CAD build for the part. Positions are in the model's coordinates, mm. Give positions to 0.01 mm unless a question says otherwise; leave off trailing zeros. Order: outer loops, then holes, each group sorted by start corner. A loop starts at its lowest first (then second) coordinate and runs counter-clockwise, first axis right, second up.
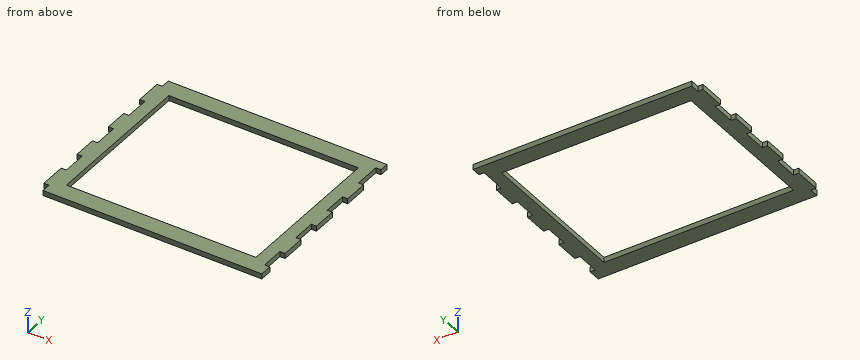
Autodesk Inventor part; units mm, degrees
ref_plane "YZ Plane" through (0, 0, 0) normal (1, 0, 0) x (0, 1, 0)
ref_plane "XZ Plane" through (0, 0, 0) normal (0, 1, 0) x (-1, 0, 0)
ref_plane "XY Plane" through (0, 0, 0) normal (0, 0, 1) x (1, 0, 0)
sketch "Boceto1" plane through (0, 0, 0) normal (0, 0, 1) x (1, 0, 0)
  line L0 (3, 3) -> (130, 3)
  line L1 (10, 103) -> (10, 13)
  line L2 (10, 13) -> (120, 13)
  line L3 (120, 13) -> (120, 103)
  line L4 (10, 103) -> (120, 103)
  line L5 (130, 113) -> (130, 106)
  line L6 (130, 106) -> (127, 107.7321)
  line L7 (130, 92.5) -> (127, 90.7679)
  line L8 (130, 65) -> (127, 63.2679)
  line L9 (130, 78.5) -> (127, 80.2321)
  line L10 (130, 10) -> (127, 8.2679)
  line L11 (130, 23.5) -> (127, 25.2321)
  line L12 (130, 51) -> (127, 52.7321)
  line L13 (130, 37.5) -> (127, 35.7679)
  line L14 (127, 107.7321) -> (127, 90.7679)
  line L15 (127, 80.2321) -> (127, 63.2679)
  line L16 (127, 52.7321) -> (127, 35.7679)
  line L17 (127, 25.2321) -> (127, 8.2679)
  line L18 (3, 113) -> (3, 106)
  line L19 (3, 106) -> (0, 107.7321)
  line L20 (3, 92.5) -> (0, 90.7679)
  line L21 (3, 65) -> (0, 63.2679)
  line L22 (3, 78.5) -> (0, 80.2321)
  line L23 (3, 10) -> (0, 8.2679)
  line L24 (3, 23.5) -> (0, 25.2321)
  line L25 (3, 37.5) -> (0, 35.7679)
  line L26 (3, 51) -> (0, 52.7321)
  line L27 (0, 107.7321) -> (0, 90.7679)
  line L28 (0, 80.2321) -> (0, 63.2679)
  line L29 (0, 52.7321) -> (0, 35.7679)
  line L30 (0, 25.2321) -> (0, 8.2679)
  line L31 (130, 113) -> (130, 106)
  line L32 (130, 92.5) -> (130, 85.5)
  line L33 (130, 113) -> (130, 106)
  line L34 (130, 113) -> (130, 106)
  line L35 (130, 92.5) -> (130, 78.5)
  line L36 (130, 92.5) -> (130, 78.5)
  line L37 (130, 65) -> (130, 58)
  line L38 (130, 65) -> (130, 51)
  line L39 (130, 37.5) -> (130, 23.5)
  line L40 (130, 10) -> (130, 3)
  line L41 (0, 8.2679) -> (0, 25.2321)
  line L42 (0, 35.7679) -> (0, 52.7321)
  line L43 (0, 63.2679) -> (0, 80.2321)
  line L44 (0, 90.7679) -> (0, 107.7321)
  line L45 (3, 113) -> (3, 106)
  line L46 (3, 92.5) -> (3, 85.5)
  line L47 (3, 113) -> (3, 106)
  line L48 (3, 113) -> (3, 106)
  line L49 (3, 92.5) -> (3, 78.5)
  line L50 (3, 92.5) -> (3, 78.5)
  line L51 (3, 65) -> (3, 58)
  line L52 (3, 65) -> (3, 51)
  line L53 (3, 37.5) -> (3, 23.5)
  line L54 (3, 10) -> (3, 3)
  line L55 (3, 113) -> (130, 113)
  line L56 (0, 107.7321) -> (3, 107.7321)
  line L57 (0, 92.5) -> (3, 92.5)
  line L58 (0, 78.5) -> (3, 78.5)
  line L59 (0, 65) -> (3, 65)
  line L60 (0, 51) -> (3, 51)
  line L61 (0, 37.5) -> (3, 37.5)
  line L62 (0, 23.5) -> (3, 23.5)
  line L63 (0, 8.2679) -> (3, 8.2679)
  line L64 (127, 107.7321) -> (130, 107.7321)
  line L65 (127, 92.5) -> (130, 92.5)
  line L66 (127, 78.5) -> (130, 78.5)
  line L67 (127, 65) -> (130, 65)
  line L68 (127, 51) -> (130, 51)
  line L69 (127, 37.5) -> (130, 37.5)
  line L70 (127, 23.5) -> (130, 23.5)
  line L71 (127, 10) -> (130, 10)
  line L72 (127, 8.2679) -> (130, 8.2679)
  point P0 (0, 0)
  point P1 (0, 58)
  point P2 (3, 3)
  point P3 (127, 99.25)
  dimension "d11" = 7
  dimension "d14" = 7
  dimension "d18" = 3
  dimension "d20" = 44.4641
  dimension "d21" = 7
  dimension "d22" = 65.5359
  dimension "d24" = 130
  dimension "d25" = 110
  dimension "d26" = 7
extrude "Extrusión1" add sketch "Boceto1" against normal blind 3 contours L54 L23 L30 L62 L53 L61 L29 L60 L52 L51 L59 L28 L58 L49 L46 L57 L27 L19 L18 L55 L5 L64 L14 L7 L32 L35 L9 L15 L8 L37 L38 L12 L16 L13 L39 L11 L17 L72 L40 L0 | L63 L23 L54 | L72 L10 L40 | L10 L17 L71 | L17 L11 L70 | L13 L16 L69 | L16 L12 L68 | L8 L15 L67 | L15 L9 L66 | L7 L14 L65 | L56 L18 L19
Item 1: Slice it at A-A (y = 21.5). Give the cut face in (x, z), and give its area (3 significant figures).
Item 2: Wall check: L1, parallel to Y at x = 74.5, z = -1.8; L2, parallel to X at y = 97, z = -0.9; L3, parallel to X at y = 61.5, z = -1.6. Give the ranges that are in metal, low to high.
Item 3: Drop flat-ended pins along their axis: pin 1 Ø1.5 at (y, z) = (14.5, -1) entering from +X; pin 2 Ø3 at (x, y) = (31, 15.5) entering from +Z; pin 3 Ø1 at (y, z) = (56.5, -0.5) entering from -X; pin 4 Ø0.9 at (x, z) = (1, -2) entering from -Y. Give the stop position or say it passes through.
Item 4: Slice it at B-B (x = 27). Give the cut face in (y, z).
A:
1. outline: (0, -3) - (10, -3) - (10, 0) - (0, 0) - close; (120, -3) - (127, -3) - (127, 0) - (120, 0) - close
1. area: 51.0 mm2
2. L1: y = 3 to 13, 103 to 113
2. L2: x = 0 to 10, 120 to 127
2. L3: x = 3 to 10, 120 to 130
3. pin 1: stops at x = 127
3. pin 2: passes through
3. pin 3: stops at x = 3
3. pin 4: stops at y = 8.27
4. outline: (3, -3) - (13, -3) - (13, 0) - (3, 0) - close; (103, -3) - (113, -3) - (113, 0) - (103, 0) - close
